Check sheet for the modelled part. Datum: model origin and axes. Units: mm. A direction names the side the tool comes from. Give positions to 0.01 mm unless a question says otherwise; leave off trailing zeros. Order: outer loops, then holes, each group sorted by start corner. A loop starts at its lowest first (then second) coordinate and runs counter-clockwise, first axis right, second up. Notation, with made-up numbers: (-32.75, 55.25) -> (10.25, 55.25) arc R25 ccw to (10.25, 94.25) -> close; hole circle Ø9 at (54, -37.5). An arc over 180 degrees is marked (long way). Write each question's results on one line, items separated by ' | '.
from build123d import *

# Parameters (mm, degrees)
SKETCH1_R           = 12.7
BOSS_EXTRUDE1_DEPTH = 36.515
SKETCH2_W           = 17.02
SKETCH2_H           = 19.05
BOSS_EXTRUDE2_DEPTH = 1.59
FILLET1_RADIUS      = 1.59
FILLET1_LENGTH      = 19.05
FILLET2_RADIUS      = 1.59
FILLET2_LENGTH      = 19.05
FILLET3_RADIUS      = 1.59
FILLET3_LENGTH      = 19.05
FILLET4_RADIUS      = 1.59
FILLET4_LENGTH      = 19.05


with BuildPart() as part:
    # Sketch1 → Boss-Extrude1 (new, symmetric)
    with BuildSketch(Plane.XY):
        Circle(SKETCH1_R)
    extrude(amount=BOSS_EXTRUDE1_DEPTH, both=True)

    # Sketch2 → Boss-Extrude2 (add, symmetric)
    # profile 1 of 2: a face of its own
    with BuildSketch(Plane(origin=(0, 0, 0), x_dir=(1, 0, 0), z_dir=(0, 1, 0))):
        with Locations((0, 46.04)):
            Rectangle(SKETCH2_W, SKETCH2_H)
        with BuildLine():
            Line((-4.365, 42.06), (-4.365, 47.62))
            ThreePointArc((-4.365, 47.62), (0, 51.985), (4.365, 47.62))
            Line((4.365, 47.62), (4.365, 42.06))
            ThreePointArc((4.365, 42.06), (0, 37.695), (-4.365, 42.06))
        make_face(mode=Mode.SUBTRACT)
    # profile 2 of 2: a face of its own
    with BuildSketch(Plane(origin=(0, 0, 0), x_dir=(1, 0, 0), z_dir=(0, 1, 0))):
        with Locations((0, -46.04)):
            Rectangle(SKETCH2_W, SKETCH2_H)
        with BuildLine():
            Line((4.365, -42.06), (4.365, -47.62))
            ThreePointArc((4.365, -47.62), (0, -51.985), (-4.365, -47.62))
            Line((-4.365, -47.62), (-4.365, -42.06))
            ThreePointArc((-4.365, -42.06), (0, -37.695), (4.365, -42.06))
        make_face(mode=Mode.SUBTRACT)
    extrude(amount=BOSS_EXTRUDE2_DEPTH, both=True)

    # Fillet1: full round fillet: the end face becomes a half cylinder, R = half its width
    fillet1_face = Plane((-8.51, 0, -46.04), x_dir=(0, 0, 1), z_dir=(-1, 0, 0))  # on the end face: x along it, z out of the body
    fillet1_slab = fillet1_face.offset(-FILLET1_RADIUS / 2) * Box(FILLET1_LENGTH, 2 * FILLET1_RADIUS, FILLET1_RADIUS, mode=Mode.PRIVATE)  # the body's end, R deep
    fillet1_round = Plane((-6.92, 0, -46.04), x_dir=(-1, 0, 0), z_dir=(0, 0, 1)) * Cylinder(FILLET1_RADIUS, FILLET1_LENGTH, mode=Mode.PRIVATE)  # its axis R under the face
    add(fillet1_slab - fillet1_round, mode=Mode.SUBTRACT)

    # Fillet2: full round fillet: the end face becomes a half cylinder, R = half its width
    fillet2_face = Plane((8.51, 0, -46.04), x_dir=(0, 0, -1), z_dir=(1, 0, 0))  # on the end face: x along it, z out of the body
    fillet2_slab = fillet2_face.offset(-FILLET2_RADIUS / 2) * Box(FILLET2_LENGTH, 2 * FILLET2_RADIUS, FILLET2_RADIUS, mode=Mode.PRIVATE)  # the body's end, R deep
    fillet2_round = Plane((6.92, 0, -46.04), x_dir=(1, 0, 0), z_dir=(0, 0, -1)) * Cylinder(FILLET2_RADIUS, FILLET2_LENGTH, mode=Mode.PRIVATE)  # its axis R under the face
    add(fillet2_slab - fillet2_round, mode=Mode.SUBTRACT)

    # Fillet3: full round fillet: the end face becomes a half cylinder, R = half its width
    fillet3_face = Plane((8.51, 0, 46.04), x_dir=(0, 0, 1), z_dir=(1, 0, 0))  # on the end face: x along it, z out of the body
    fillet3_slab = fillet3_face.offset(-FILLET3_RADIUS / 2) * Box(FILLET3_LENGTH, 2 * FILLET3_RADIUS, FILLET3_RADIUS, mode=Mode.PRIVATE)  # the body's end, R deep
    fillet3_round = Plane((6.92, 0, 46.04), x_dir=(1, 0, 0), z_dir=(0, 0, 1)) * Cylinder(FILLET3_RADIUS, FILLET3_LENGTH, mode=Mode.PRIVATE)  # its axis R under the face
    add(fillet3_slab - fillet3_round, mode=Mode.SUBTRACT)

    # Fillet4: full round fillet: the end face becomes a half cylinder, R = half its width
    fillet4_face = Plane((-8.51, 0, 46.04), x_dir=(0, 0, -1), z_dir=(-1, 0, 0))  # on the end face: x along it, z out of the body
    fillet4_slab = fillet4_face.offset(-FILLET4_RADIUS / 2) * Box(FILLET4_LENGTH, 2 * FILLET4_RADIUS, FILLET4_RADIUS, mode=Mode.PRIVATE)  # the body's end, R deep
    fillet4_round = Plane((-6.92, 0, 46.04), x_dir=(-1, 0, 0), z_dir=(0, 0, -1)) * Cylinder(FILLET4_RADIUS, FILLET4_LENGTH, mode=Mode.PRIVATE)  # its axis R under the face
    add(fillet4_slab - fillet4_round, mode=Mode.SUBTRACT)


solid = part.part
1. Mould release check, pull along Z, two halves, no side actions. Record for faces 1 (the cylindrical face through (-8.51, 0.03, -45.91)), 2 (the flat face through (0, 0, -55.565)), 3 (the cylindrical face through (-0.096, 0.022, 37.696)): +Z half, -Z half, draft (parallel to the pull), parting line (faces both ways), or undercut.
Verdict:
face 1: draft | face 2: -Z half | face 3: undercut
2. Gauge pin test, flat ends, axial feed: pin 1 Ø10 at (y, z) = (1.5, 35.5) entering from +X; pin 2 Ø7 at (x, z) = (2, 43.5) entering from +Y; pin 3 Ø7 at (x, z) = (0, -42.5) entering from +Y; pin 4 Ø8 at (x, z) = (6, 2) entering from -Y. Record the tip position at first contact, or that the pin passes through.
Verdict:
pin 1: stops at x = 12.7 | pin 2: stops at y = 1.59 | pin 3: passes through | pin 4: stops at y = -12.54
3. Access from +Z, -Z, +X, -X, +Y, -Y to the whole of each face (thin tool, end or side, straight path). Record for faces 4 (the cylindrical face through (0.096, 0.022, 51.984)), 5 (the cylindrical face through (8.51, -0.03, 46.17)), 6 (the flat face through (-5, -1.59, -46)), 7 (the cylindrical face through (-8.51, -0.03, 45.91)).
Verdict:
face 4: +Y, -Y | face 5: +Z, +X | face 6: -Z, +X, -X, -Y | face 7: +Z, -X
4. Section check D-D on x = -11. Record the cut outline in (y, z) (3 decimals), then the cut area to 3 significant figures.
Verdict:
outline: (-6.347, -36.515) -> (6.347, -36.515) -> (6.347, 36.515) -> (-6.347, 36.515) -> close | area: 927 mm^2
5. Section check B-B on z = 13. Record the cut outline in (x, y).
Verdict:
outline: circle Ø25.4 at (0, 0)
6. Section check A-A on x = 0. Record the cut outline in (y, z) (3 decimals), then the cut area to 3 significant figures.
Verdict:
outline: (-12.7, -36.515) -> (-1.59, -36.515) -> (-1.59, -37.695) -> (1.59, -37.695) -> (1.59, -36.515) -> (12.7, -36.515) -> (12.7, 36.515) -> (1.59, 36.515) -> (1.59, 37.695) -> (-1.59, 37.695) -> (-1.59, 36.515) -> (-12.7, 36.515) -> close; (-1.59, -55.565) -> (1.59, -55.565) -> (1.59, -51.985) -> (-1.59, -51.985) -> close; (-1.59, 51.985) -> (1.59, 51.985) -> (1.59, 55.565) -> (-1.59, 55.565) -> close | area: 1,890 mm^2
7. Section check C-C on y = -6.75. Record the cut outline in (x, z) (3 decimals).
Verdict:
outline: (-10.758, -36.515) -> (10.758, -36.515) -> (10.758, 36.515) -> (-10.758, 36.515) -> close
8. Material ranges on probe 1 along Z at (x, y) = (1, 1.25) (3 decimals); probe 2 along Z at (x, y) = (-2, 10.5) (3 decimals); probe 3 along X at (y, z) = (0.5, -30.5), recorded low to high. Write a range as from..to.
Verdict:
probe 1: z = -55.565..-51.869, -37.811..37.811, 51.869..55.565 | probe 2: z = -36.515..36.515 | probe 3: x = -12.69..12.69
